```python
from build123d import *

# Parameters (mm, degrees)
ESQUISSE1_R                  = 6
CYLINDRE_EXTERIEUR_DEPTH     = 28
TENON_DEPTH                  = 10
TENON_DEPTH_BACK             = 10
ESQUISSE3_W                  = 6
ESQUISSE3_H                  = 7
ESQUISSE3_H_2                = 9
CHANFREIN1_SIZE              = 0.5
PER_AGE1_D                   = 4.5
PER_AGE1_DEPTH               = 18.5
PER_AGE1_TIP                 = 1.351936393
ENL_V_MAT_EXTRU_2_DEPTH      = 10
ENL_V_MAT_EXTRU_2_DEPTH_BACK = 30.257477677
ESQUISSE6_R                  = 2


with BuildPart() as part:
    # Esquisse1 → Cylindre exterieur (new body)
    with BuildSketch(Plane.XY):
        with Locations(Location((0, 0, 0), (0, 0, 245.375681648))):
            Circle(ESQUISSE1_R)
    extrude(amount=CYLINDRE_EXTERIEUR_DEPTH)

    # Esquisse3 → Tenon (cut, two sides: drawn at the far end of the back side and taken through both)
    with BuildSketch(Plane(origin=(0, 0, 0), x_dir=(1, 0, 0), z_dir=(0, 1, 0)).offset(-TENON_DEPTH_BACK)):
        with Locations((5.5, -2.5)):
            Rectangle(ESQUISSE3_W, ESQUISSE3_H)
        with Locations((-5.5, -1.5)):
            Rectangle(ESQUISSE3_W, ESQUISSE3_H_2)
    extrude(amount=TENON_DEPTH + TENON_DEPTH_BACK, mode=Mode.SUBTRACT)

    # Chanfrein1
    chanfrein1_edges = [part.edges().sort_by_distance(p)[0] for p in [
        (0, -6, 0),
        (0, 6, 0),
    ]]
    chamfer(chanfrein1_edges, length=CHANFREIN1_SIZE)

    # Perçage1
    with Locations(Plane.XY.offset(28)):
        with Locations((0, 0)):
            Hole(PER_AGE1_D / 2, depth=PER_AGE1_DEPTH)
            with Locations((0, 0, -(PER_AGE1_DEPTH + PER_AGE1_TIP / 2))):  # 118° drill point
                Cone(0, PER_AGE1_D / 2, PER_AGE1_TIP, mode=Mode.SUBTRACT)

    # Esquisse6 → Enlèv. mat.-Extru.2 (cut, two sides: drawn at the far end of the back side and taken through both)
    with BuildSketch(Plane(origin=(0, 0, 0), x_dir=(0, 0, -1), z_dir=(1, 0, 0)).offset(-ENL_V_MAT_EXTRU_2_DEPTH_BACK)):
        with Locations((-21, 0)):
            Circle(ESQUISSE6_R)
    extrude(amount=ENL_V_MAT_EXTRU_2_DEPTH + ENL_V_MAT_EXTRU_2_DEPTH_BACK, mode=Mode.SUBTRACT)


solid = part.part
```
Read the model definition and answer for the solid it produces. Units are mm, in the model's axes. A direction names the side the tool comes from. Round coordinates to 2 decimals unless told otherwise and drop trailing zeros. Write each loop counter-clockwise with the first axis right and the second up, starting at its lowest first coordinate (ties: lowest second). Pieces come first, ordered by that corner, then holes. Notation, with made-up numbers: (12, -30.5) -> (56, -30.5) arc R13 ccw to (56, -17.5) -> close; hole circle Ø2 at (-33.75, -19). An arc over 180 degrees is marked (long way). Answer in a Markdown table with one row per item. Add a question column.
1) Determine the mould class of faces 4 (the face through (-4.8, 3.6, 17.1)), 5 (the face through (-1, -2.4, 28)), 6 (the face through (0.37, 0.12, 8.38)) for opening direction Y: pulls with the +Y half, pulls with the -Y half, needs draft (parallel to the pull), parting line crosses it, or undercut.
2) Find section B-B, the plane x = -3. Determine the outline of the cut face in (y, z).
3) Consider line 1 (X direction, y = 0, z = 17.5); line 2 (Y direction, x = 4.9, z = 21). Determine where each line is inside the solid, lowest interval first.
4) Given P1, Ø1.8, axis at x = 3.5, y = -2.5, coming from the -Z side; P2, Ø4, axis at x = 3.5, z = 17.5, coming from the +Y side; P3, Ø1, axis at y = -3.5, z = 22, coming from the +X side, each flat-ended and moving along its own axis, determine where each tip first touches the part or whether it passes through.
5) Find section C-C, the plane y = 2.75. Determine the outline of the cut face in (x, z), and give its area (3 significant figures).
6) Find section D-D, the plane z = 4.75. Determine the outline of the cut face in (x, y), and give its area (3 significant figures).
7) Find section A-A, the plane z = 22.5. Determine the outline of the cut face in (x, y).
8) Which of the six approach directions +Z, -Z, +X, -X, +Y, -Y give full straight-line access (tool end or side, diameter ignored) to faces 1 (the face through (1.786, -1.369, 18.62)), 2 (the face through (-2.5, 0, 3)), 3 (the face through (2.5, 0, 3))?
Findings below:
| question | item | result |
|---|---|---|
| 1 | face 4 | parting line crosses it |
| 1 | face 5 | needs draft |
| 1 | face 6 | undercut |
| 2 | outline | (-5.2, 6) -> (5.2, 6) -> (5.2, 28) -> (-5.2, 28) -> close; hole circle Ø4 at (0, 21) |
| 3 | line 1 | -6 to -2.25, 2.25 to 6 |
| 3 | line 2 | -3.46 to -2, 2 to 3.46 |
| 4 | P1 | z = 6 |
| 4 | P2 | y = 5.81 |
| 4 | P3 | x = 5.2 |
| 5 | outline | (-5.33, 6) -> (-2.5, 6) -> (-2.5, 0) -> (2.5, 0) -> (2.5, 6) -> (5.33, 6) -> (5.33, 28) -> (-5.33, 28) -> close |
| 5 | area | 265 mm² |
| 6 | outline | (-2.5, -5.45) arc R6 ccw to (2.5, -5.45) -> (2.5, 5.45) arc R6 ccw to (-2.5, 5.45) -> close |
| 6 | area | 58.2 mm² |
| 7 | outline | (-5.85, -1.32) arc R6 ccw to (5.85, -1.32) -> (1.82, -1.32) arc R2.25 cw to (-1.82, -1.32) -> close; (-5.85, 1.32) -> (-1.82, 1.32) arc R2.25 cw to (1.82, 1.32) -> (5.85, 1.32) arc R6 ccw to start |
| 8 | face 1 | +Z |
| 8 | face 2 | -Z, -X, +Y, -Y |
| 8 | face 3 | -Z, +X, +Y, -Y |
